Check sheet for the modelled part. Datum: model origin and axes. Units: mm. Round coordinates to 2 decimals unless told otherwise and drop trailing zeros. Order: outer loops, then holes, each group sorted by start corner. A loop starts at its lowest first (then second) coordinate and runs counter-clockwise, first axis right, second up.
```python
from build123d import *

# Parameters (mm, degrees)
ESQUISSE1_W                         = 45
ESQUISSE1_H                         = 26
BOSS_EXTRU_1_DEPTH                  = 20
ENL_V_MAT_EXTRU_1_REACH             = 22
ESQUISSE3_R                         = 5
ENL_V_MAT_EXTRU_1_DIRECTION_2_DEPTH = 1
TROU_TARAUD_M101_D                  = 8.5
TROU_TARAUD_M101_DEPTH              = 26


with BuildPart() as part:
    # Esquisse1 → Boss.-Extru.1 (new body)
    with BuildSketch(Plane.XY):
        with Locations((-22.5, 13)):
            Rectangle(ESQUISSE1_W, ESQUISSE1_H)
    extrude(amount=BOSS_EXTRU_1_DEPTH)

    # Esquisse3 → Enlèv. mat.-Extru.1 (cut, up to next)
    with BuildSketch(Plane(origin=(0, 0, 0), x_dir=(-1, 0, 0), z_dir=(0, 0, -1)), mode=Mode.PRIVATE) as enl_v_mat_extru_1_sk1:
        with Locations(Location((22, 13, 0), (0, 0, 180))):  # turned: the seam where the file's is
            Circle(ESQUISSE3_R)
    enl_v_mat_extru_1_tool1 = extrude(enl_v_mat_extru_1_sk1.sketch, amount=-ENL_V_MAT_EXTRU_1_REACH, mode=Mode.PRIVATE) & part.part
    add(enl_v_mat_extru_1_tool1.solids().sort_by_distance((-22, 13, 0))[0], mode=Mode.SUBTRACT)

    # Esquisse3 → Enlèv. mat.-Extru.1 direction 2 (cut)
    with BuildSketch(Plane(origin=(0, 0, 0), x_dir=(-1, 0, 0), z_dir=(0, 0, -1))):
        with Locations(Location((22, 13, 0), (0, 0, 180))):  # turned: the seam where the file's is
            Circle(ESQUISSE3_R)
    extrude(amount=ENL_V_MAT_EXTRU_1_DIRECTION_2_DEPTH, mode=Mode.SUBTRACT)

    # Trou taraudé M101
    with Locations(Plane(origin=(0, 26, 0), x_dir=(1, 0, 0), z_dir=(0, 1, 0))):
        with Locations((-8, -10)):
            Hole(TROU_TARAUD_M101_D / 2, depth=TROU_TARAUD_M101_DEPTH)


solid = part.part
```
Item 1: Sectioned sample at B-B (y = 13). Record the cut outline in (x, z).
Answer:
outline: (-45, 0) - (-27, 0) - (-27, 20) - (-45, 20) - close; (-17, 0) - (0, 0) - (0, 20) - (-17, 20) - close; hole circle Ø8.5 at (-8, 10)
Item 2: Sectioned sample at C-C (x = -22). Record the cut outline in (y, z).
Answer:
outline: (0, 0) - (8, 0) - (8, 20) - (0, 20) - close; (18, 0) - (26, 0) - (26, 20) - (18, 20) - close
Item 3: Sectioned sample at D-D (x = -8). Record the cut outline in (y, z), and give its area (3 significant figures).
Answer:
outline: (0, 0) - (26, 0) - (26, 5.75) - (0, 5.75) - close; (0, 14.25) - (26, 14.25) - (26, 20) - (0, 20) - close
area: 299 mm2
Item 4: Release check for a two-part mould opening along Y. For faces 1 (the flat face through (-23, 0, 10)), 2 (the cylindrical face through (-27, 13, 10)), 3 (the flat face through (-45, 13, 10)), 4 (the flat face through (-23, 26, 10)) record: released by +Y, released by -Y, zero draft, split by the parting line, or undercut.
Answer:
face 1: released by -Y
face 2: undercut
face 3: zero draft
face 4: released by +Y
Item 5: Scan lines: line 1 along Z through (x, y) = (-8, 18); line 2 along X through (y, z) = (13, 15.5); line 3 along Y through (x, z) = (-22, 2). Record each from-to range of solid material in increasing order.
Answer:
line 1: z = 0 to 5.75, 14.25 to 20
line 2: x = -45 to -27, -17 to 0
line 3: y = 0 to 8, 18 to 26
Item 6: Sectioned sample at A-A (z = 13.75). Record the cut outline in (x, y).
Answer:
outline: (-45, 0) - (-10, 0) - (-10, 26) - (-45, 26) - close; (-6, 0) - (0, 0) - (0, 26) - (-6, 26) - close; hole circle Ø10 at (-22, 13)
